```python
from build123d import *

# Parameters (mm, degrees)
CYLINDER020_R     = 14
CYLINDER020_DEPTH = 5
CYLINDER018_R     = 20
CYLINDER018_DEPTH = 3
CYLINDER019_R     = 17
CYLINDER019_DEPTH = 5


with BuildPart() as cylinder004:
    # Cylinder020 → Cylinder020 (new body)
    with BuildSketch(Plane.XY):
        Circle(CYLINDER020_R)
    extrude(amount=CYLINDER020_DEPTH)


with BuildPart() as cylinder002:
    # Cylinder018 → Cylinder018 (new body)
    with BuildSketch(Plane.XY):
        Circle(CYLINDER018_R)
    extrude(amount=CYLINDER018_DEPTH)


with BuildPart() as cut031:
    # Cylinder019 → Cylinder019 (new body)
    with BuildSketch(Plane.XY):
        Circle(CYLINDER019_R)
    extrude(amount=CYLINDER019_DEPTH)

    # Fusion024: union Cylinder002
    add(cylinder002.part)

    # Cut031: cut Cylinder004
    add(cylinder004.part, mode=Mode.SUBTRACT)


with BuildPart() as cut031_1:
    # Cut031 placement: moved
    add(cut031.part.moved(Location((0, 0, 10))))


solid = cut031_1.part
```
Here's how the part is built. I have some questions about the finished solid (model axes, mm). A direction names the side the tool comes from. Round coordinates to 2 decimals unless told otherwise and drop trailing zeros. Loops run counter-clockwise (first coordinate to the right, second up) from the corner with the lowest first, then second, coordinate; pieces in that order, holes last. Notation, with made-up numbers: (72, 8.5) -> (82, 8.5) arc R35 cw to (82, 44.5) -> close; hole circle Ø3 at (-10, 15). An arc over 180 degrees is marked (long way). Answer as CSV lines item,"result". Start each with the question number.
1. For faces 1 (the face through (-4.336, -19.524, 11.479)), 2 (the face through (-9, -15, 13)), which set-ups out of +Z, -Z, +X, -X, +Y, -Y let a thin tool reach every point of the face, with its end or its side?
2. I'm going to push flat-ended pins straight in: P1, Ø1.5, axis at x = 2.5, z = 11, coming from the +Y side; P2, Ø3, axis at x = -6.5, z = 12.5, coming from the +Y side; P3, Ø4, axis at x = 3.5, y = -10.5, coming from the +Z side; P4, Ø2, axis at x = 5, z = 12, coming from the +Y side. Where does each tip first touch, or does it pass through?
3. I need wall thicknesses on probe 1 along Y at (x, z) = (0, 12.95); probe 2 along X at (y, z) = (-5, 10.3); probe 3 along X at (y, z) = (-10.5, 13.2). Which ranges of each line are inside material? Lowest first, please. Write a range as from..to.
4. Imagine slicing it at A-A on x = 0. Write out the boundary of the cut face in (y, z).
5. Imagine slicing it at C-C on z = 12.3. Write out the boundary of the cut face in (x, y), plus the area to 3 significant figures.
6. If we mould it in two halves opening along Y, with no side actions, what happens to faces 3 (the face through (9.139, 14.334, 13.986)), 4 (the face through (-14, -4, 10)), 5 (the face through (12.932, -5.362, 12.465))? For each: pulls with the +Y half, pulls with the -Y half, needs draft (parallel to the pull), parting line crosses it, or undercut.
Solution:
1,face 1,"+Z, -Z"
1,face 2,"+Z"
2,P1,"y = 19.92"
2,P2,"y = 19.36"
2,P3,"through"
2,P4,"y = 19.6"
3,probe 1,"-20..-14, 14..20"
3,probe 2,"-19.36..-13.08, 13.08..19.36"
3,probe 3,"-13.37..-9.26, 9.26..13.37"
4,outline,"(-20, 10) -> (-14, 10) -> (-14, 15) -> (-17, 15) -> (-17, 13) -> (-20, 13) -> close; (14, 10) -> (20, 10) -> (20, 13) -> (17, 13) -> (17, 15) -> (14, 15) -> close"
5,outline,"circle Ø40 at (0, 0); hole circle Ø28 at (0, 0)"
5,area,"641 mm²"
6,face 3,"parting line crosses it"
6,face 4,"needs draft"
6,face 5,"undercut"
